Input: part model. Units: mm. Frame: model coordinates. Face numbers are marked on the shaded views. Round coordinates to 2 decimals unless told otherwise and drop trailing zeros. Loops run counter-clockwise (first coordinate to the right, second up) from the corner with the lowest first, then second, coordinate; pieces in that order, holes last. Notation, with made-up numbers: M -18.5,84.25 L -2.5,84.25 A5 ccw -2.5,88.25 Z; hole C 86.5,28 d10. An arc over 180 degrees is marked long. Put each result on its own line as item: value. Start each with the question number.
1) Pin query (flat end, axial travel): pin 1 (8 mm diameter, centred on x = 637, y = 7, fed in from +Z); pin 2 (5 mm diameter, centred on y = 3, z = -423.5, fed in from +X); pin 3 (11 mm diameter, centred on x = 512.5, y = 7, fed in from -Z). Return the tip coordinate at first contact, or that it passes through.
2) Section D-D on y = 51.5. Output: boundary loops of the cut face in (x, z).
3) Section A-A on z = -270.5. Output: boundary loops of the cut face in (x, y), plus the area to 3 significant figures.
4) Section B-B on x = 500. Output: boundary loops of the cut face in (y, z).
5) Section C-C on x = 184.5. Output: boundary loops of the cut face in (y, z).
6) Line query: probe 1 along Y at (x, z) = (239, -161.5); probe 2 along X at (y, z) = (6, -186.5); probe 3 along Y at (x, z) = (361, 8.5). Output: solid intervals per line, ascending.
7) Draft query along Y for the marked faces 1, 2 and 3. Return one class per face: +Y half, -Y half, draft (parallel to the pull), parting line (faces both ways), or undercut.
Autodesk Inventor part; units mm, degrees
ref_plane "YZ Plane" through (0, 0, 0) normal (1, 0, 0) x (0, 1, 0)
ref_plane "XZ Plane" through (0, 0, 0) normal (0, 1, 0) x (-1, 0, 0)
ref_plane "XY Plane" through (0, 0, 0) normal (0, 0, 1) x (1, 0, 0)
sketch "Sketch1" plane through (0, 0, 0) normal (0, 1, 0) x (-1, 0, 0)
  line L0 (0, 0) -> (-853.55, 0)
  line L1 (-853.55, 0) -> (-853.55, -707.1)
  line L2 (-853.55, -707.1) -> (0, -707.1)
  line L3 (0, -707.1) -> (0, 0)
  dimension "d0" = 853.55
  dimension "d1" = 707.1
extrude "Extrusion1" add sketch "Sketch1" along normal blind 10
ref_plane "Work Plane4" through (500, 0, 0) normal (1, 0, 0) x (0, 0, -1)
ref_plane "Work Plane3" through (146.45, 0, 0) normal (1, 0, 0) x (0, 0, -1)
ref_plane "Work Plane2" through (853.55, 0, -353.55) normal (0, 0, -1) x (-1, 0, 0)
ref_plane "Work Plane5" through (500, 0, -353.55) normal (0.7071, 0, -0.7071) x (0, 1, 0)
ref_plane "Work Plane6" through (500, 0, -353.55) normal (0.7071, 0, 0.7071) x (0, -1, 0)
sketch "Sketch2" plane through (0, 10, 0) normal (0, 1, 0) x (1, 0, 0)
  line L0 (500, 848.52) -> (500, -141.42)
  line L1 (1009.615, 863.165) -> (-82.84, -229.29)
  line L2 (-170.71, 353.55) -> (1024.26, 353.55)
  line L3 (0, 0) -> (853.55, 0)
  line L4 (853.55, 0) -> (853.55, 707.1)
  line L5 (853.55, 707.1) -> (0, 707.1)
  line L6 (0, 707.1) -> (0, 0)
  circle A0 centre (500, 353.55) radius 37.5
  dimension "d5" = 75
extrude "Extrusion2" add sketch "Sketch2" along normal blind 85 contours A0 L1 L0 | L0 L2 A0 | L2 A0 L0 | L0 A0 L1 | L1 A0 L2 | L1 A0 L2
sketch "Sketch3" plane through (500, 95, -353.55) normal (0, 1, 0) x (1, 0, 0)
  circle A0 centre (0, 0) radius 500
  point P0 (-500, -353.55)
  dimension "d8" = 1000
extrude "Extrusion3" add sketch "Sketch3" along normal blind 10
properties part number "rotating_turntable"
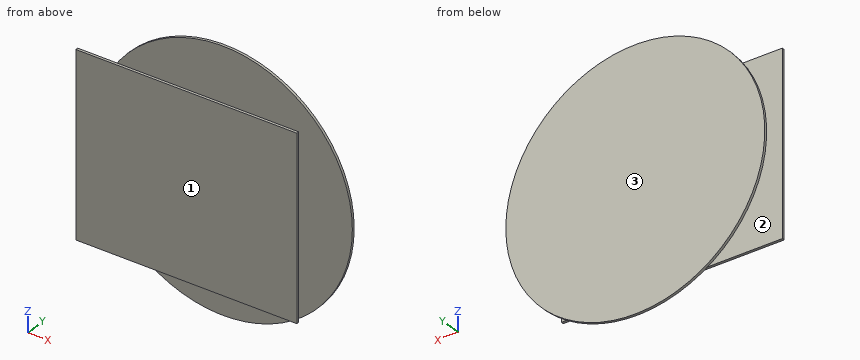
Geometry results:
1. pin 1: stops at z = 0
1. pin 2: stops at x = 853.55
1. pin 3: stops at z = -707.1
2. outline: C 500,-353.55 d75
3. outline: M 0,0 L 853.55,0 L 853.55,10 L 0,10 Z; M 6.95,95 L 993.05,95 L 993.05,105 L 6.95,105 Z
3. area: 18,400 mm²
4. outline: M 0,-707.1 L 10,-707.1 L 10,-391.05 L 95,-391.05 L 95,-853.55 L 105,-853.55 L 105,146.45 L 95,146.45 L 95,-316.05 L 10,-316.05 L 10,0 L 0,0 Z
5. outline: M 0,-707.1 L 10,-707.1 L 10,0 L 0,0 Z; M 95,-741.44 L 105,-741.44 L 105,34.34 L 95,34.34 Z
6. probe 1: y = 0 to 10, 95 to 105
6. probe 2: x = 0 to 853.55
6. probe 3: y = 95 to 105
7. face 1: -Y half
7. face 2: undercut
7. face 3: +Y half
